Verification items for the finished model (mm, model axes). Face numbers are marked on the shaded views. A direction names the side the tool comes from. Give positions to 0.01 mm unless a question says otherwise; leave off trailing zeros. Write each loop counter-clockwise with the first axis right and the second up, starting at its lowest first coordinate (ties: lowest second). Pieces come first, ordered by that corner, then holes.
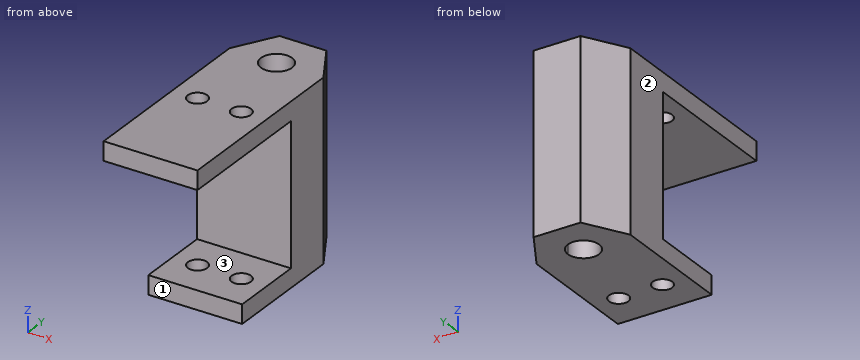
from build123d import *

# Parameters (mm, degrees)
BOSS_EXTRUDE1_DEPTH   = 28.5
SKETCH2_W             = 15
SKETCH2_H             = 3
BOSS_EXTRUDE2_DEPTH   = 23
SKETCH2_3_W           = 15
SKETCH2_3_H           = 3
BOSS_EXTRUDE3_DEPTH   = 12
SKETCH5_R             = 1.55
CUT_EXTRUDE1_DEPTH    = 29.5
M6_TAPPED_HOLE1_D     = 5
M6_TAPPED_HOLE1_DEPTH = 8
M6_TAPPED_HOLE1_TIP   = 1.502151548
M6_TAPPED_HOLE2_D     = 5
M6_TAPPED_HOLE2_DEPTH = 6
M6_TAPPED_HOLE2_TIP   = 1.502151548
SKETCH6_R             = 2.5
CUT_EXTRUDE2_DEPTH    = 29.5


with BuildPart() as part:
    # Sketch1 → Boss-Extrude1 (new body)
    with BuildSketch(Plane.XY):
        Polygon((-7.5, 0), (-7.5, -8), (7.5, -8), (7.5, 0), (3.75, 6.495190528), (-3.75, 6.495190528), align=None)
    extrude(amount=BOSS_EXTRUDE1_DEPTH)

    # Sketch2 → Boss-Extrude2 (add)
    with BuildSketch(Plane.XZ.offset(8)):
        with Locations((0, 27)):
            Rectangle(SKETCH2_W, SKETCH2_H)
    extrude(amount=BOSS_EXTRUDE2_DEPTH)

    # Sketch2<3> → Boss-Extrude3 (add)
    with BuildSketch(Plane.XZ.offset(8)):
        with Locations((0, 1.5)):
            Rectangle(SKETCH2_3_W, SKETCH2_3_H)
    extrude(amount=BOSS_EXTRUDE3_DEPTH)

    # Sketch5 → Cut-Extrude1 (cut, through all)
    with BuildSketch(Plane(origin=(0, 0, 0), x_dir=(-1, 0, 0), z_dir=(0, 0, -1))):
        with Locations((-3.5, -14.05)):
            Circle(SKETCH5_R)
        with Locations((3.5, -14.05)):
            Circle(SKETCH5_R)
    extrude(amount=-CUT_EXTRUDE1_DEPTH, mode=Mode.SUBTRACT)

    # M6 Tapped Hole1
    with Locations(Plane(origin=(0, 0, 0), x_dir=(-1, 0, 0), z_dir=(0, 0, -1))):
        with Locations((0, 0)):
            Hole(M6_TAPPED_HOLE1_D / 2, depth=M6_TAPPED_HOLE1_DEPTH)
            with Locations((0, 0, -(M6_TAPPED_HOLE1_DEPTH + M6_TAPPED_HOLE1_TIP / 2))):  # 118° drill point
                Cone(0, M6_TAPPED_HOLE1_D / 2, M6_TAPPED_HOLE1_TIP, mode=Mode.SUBTRACT)

    # M6 Tapped Hole2
    with Locations(Plane.XY.offset(28.5)):
        with Locations((0, 0)):
            Hole(M6_TAPPED_HOLE2_D / 2, depth=M6_TAPPED_HOLE2_DEPTH)
            with Locations((0, 0, -(M6_TAPPED_HOLE2_DEPTH + M6_TAPPED_HOLE2_TIP / 2))):  # 118° drill point
                Cone(0, M6_TAPPED_HOLE2_D / 2, M6_TAPPED_HOLE2_TIP, mode=Mode.SUBTRACT)

    # Sketch6 → Cut-Extrude2 (cut, through all)
    with BuildSketch(Plane(origin=(0, 0, 0), x_dir=(-1, 0, 0), z_dir=(0, 0, -1))):
        Circle(SKETCH6_R)
    extrude(amount=-CUT_EXTRUDE2_DEPTH, mode=Mode.SUBTRACT)


solid = part.part
Item 1: Sectioned sample at A-A on x = 0. Record the cut outline in (y, z), then the cut area to 3 significant figures.
Answer key:
outline: (-31, 25.5) - (-8, 25.5) - (-8, 3) - (-20, 3) - (-20, 0) - (-2.5, 0) - (-2.5, 28.5) - (-31, 28.5) - close; (2.5, 0) - (6.5, 0) - (6.5, 28.5) - (2.5, 28.5) - close
area: 376 mm2
Item 2: Scan lines: line 1 along Y through (x, z) = (0, 27); line 2 along Z through (x, y) = (-4.5, -9); line 3 along Y through (x, z) = (-3.5, 1.8). Record each from-to range of solid material in increasing order.
Answer key:
line 1: y = -31 to -2.5, 2.5 to 6.5
line 2: z = 0 to 3, 25.5 to 28.5
line 3: y = -20 to -15.6, -12.5 to 6.5
Item 3: Sectioned sample at C-C on z = 6.75. Record the cut outline in (x, y).
Answer key:
outline: (-7.5, -8) - (7.5, -8) - (7.5, 0) - (3.75, 6.5) - (-3.75, 6.5) - (-7.5, 0) - close; hole circle Ø5 at (0, 0)
Item 4: Sectioned sample at D-D on x = -3. Record the cut outline in (y, z), then the cut area to 3 significant figures.
Answer key:
outline: (-31, 25.5) - (-15.52, 25.5) - (-15.52, 28.5) - (-31, 28.5) - close; (-20, 0) - (-15.52, 0) - (-15.52, 3) - (-20, 3) - close; (-12.58, 0) - (6.5, 0) - (6.5, 28.5) - (-12.58, 28.5) - (-12.58, 25.5) - (-8, 25.5) - (-8, 3) - (-12.58, 3) - close
area: 501 mm2
Item 5: Set-up check for the marked faces 1, 2 and 3: record each of +Z, -Z, +X, -X, +Y, -Y from which the full face is reachable in a straight line by a thin tool's end or side.
Answer key:
face 1: -Z, +X, -X, -Y
face 2: +Z, -Z, -X, +Y, -Y
face 3: +X, -X, -Y
Item 6: Depth check by flat-ended pin: pin 1 (4.5 mm diameter, centred on x = -2, z = 10, fed in from -Y); pin 2 (0.9 mm diameter, centred on x = 1, z = 2, fed in from -Y). Enter the tip coordinate at first touch or a pass-through.
Answer key:
pin 1: stops at y = -8
pin 2: stops at y = -20
Item 7: Sectioned sample at B-B on y = -14.05. Record the cut outline in (x, z), then the cut area to 3 significant figures.
Answer key:
outline: (-7.5, 0) - (-5.05, 0) - (-5.05, 3) - (-7.5, 3) - close; (-7.5, 25.5) - (-5.05, 25.5) - (-5.05, 28.5) - (-7.5, 28.5) - close; (-1.95, 0) - (1.95, 0) - (1.95, 3) - (-1.95, 3) - close; (-1.95, 25.5) - (1.95, 25.5) - (1.95, 28.5) - (-1.95, 28.5) - close; (5.05, 0) - (7.5, 0) - (7.5, 3) - (5.05, 3) - close; (5.05, 25.5) - (7.5, 25.5) - (7.5, 28.5) - (5.05, 28.5) - close
area: 52.8 mm2
